Can you work these out from the model? Positions are in its coordinate system, mm. A direction names the side the tool comes from. Give positions to 0.01 mm unless a question says otherwise; leave off trailing zeros. Order: outer loops, then holes, each group sorted by start corner. A loop starts at its lowest first (then second) coordinate and runs counter-clockwise, first axis right, second up. Notation, with made-up numbers: (45.25, 19) - (93.25, 19) arc R32 cw to (93.25, 53) - close; hole circle Ø3 at (9.5, 52). An arc over 180 degrees is marked (long way). Return JSON: item names as keys, results as strings.
```python
from build123d import *

# Parameters (mm, degrees)
F0_W     = 1.4632290646
F0_H     = 3.2
F0_W_2   = 1.9813749596
F1_DEPTH = 2.4
F2_R     = 3.6
F3_R     = 0.4
F4_SIZE  = 0.4


with BuildPart() as f1:
    # F0 (on Top) → F1 (new body)
    with BuildSketch(Plane.XY):
        with BuildLine():
            Line((-1.6, 0), (1.6, 0))
            ThreePointArc((1.6, 0), (0, 1.6), (-1.6, 0))
        make_face()
        with BuildLine():
            Line((1.6, -27.8004167259), (1.6, 0))
            ThreePointArc((1.6, 0), (0, -1.6), (-1.6, 0))
            Line((-1.6, 0), (-1.6, -16.8))
            Line((-1.6, -16.8), (-1.6, -20))
            Line((-1.6, -20), (-1.6, -40))
            Line((-1.6, -40), (1.6, -40))
            Line((1.6, -40), (1.6, -31.0004167259))
            Line((1.6, -31.0004167259), (1.6, -27.8004167259))
        make_face()
        with BuildLine():
            ThreePointArc((-1.6, 0), (0, -1.6), (1.6, 0))
            Line((1.6, 0), (-1.6, 0))
        make_face()
        with Locations((2.3316145323, -29.4004167259)):
            Rectangle(F0_W, F0_H)
        with Locations((-2.5906874798, -18.4)):
            Rectangle(F0_W_2, F0_H)
        with BuildLine():
            Line((3.0632290646, -12.50463631), (3.0632290646, -27.8004167259))
            Line((3.0632290646, -27.8004167259), (3.0632290646, -31.0004167259))
            Line((3.0632290646, -31.0004167259), (6.2632290646, -31.0004167259))
            Line((6.2632290646, -31.0004167259), (6.2632290646, -12.50463631))
            ThreePointArc((6.2632290646, -12.50463631), (4.6632290646, -14.10463631), (3.0632290646, -12.50463631))
        make_face()
        with BuildLine():
            Line((-3.5813749596, -20), (-3.5813749596, -16.8))
            Line((-3.5813749596, -16.8), (-3.5813749596, -8.7620876729))
            ThreePointArc((-3.5813749596, -8.7620876729), (-5.1813749596, -10.3620876729), (-6.7813749596, -8.7620876729))
            Line((-6.7813749596, -8.7620876729), (-6.7813749596, -20))
            Line((-6.7813749596, -20), (-3.5813749596, -20))
        make_face()
        with BuildLine():
            ThreePointArc((6.2632290646, -12.50463631), (4.6632290646, -10.90463631), (3.0632290646, -12.50463631))
            Line((3.0632290646, -12.50463631), (6.2632290646, -12.50463631))
        make_face()
        with BuildLine():
            Line((6.2632290646, -12.50463631), (3.0632290646, -12.50463631))
            ThreePointArc((3.0632290646, -12.50463631), (4.6632290646, -14.10463631), (6.2632290646, -12.50463631))
        make_face()
        with BuildLine():
            ThreePointArc((-6.7813749596, -8.7620876729), (-5.1813749596, -10.3620876729), (-3.5813749596, -8.7620876729))
            Line((-3.5813749596, -8.7620876729), (-6.7813749596, -8.7620876729))
        make_face()
        with BuildLine():
            Line((-6.7813749596, -8.7620876729), (-3.5813749596, -8.7620876729))
            ThreePointArc((-3.5813749596, -8.7620876729), (-5.1813749596, -7.1620876729), (-6.7813749596, -8.7620876729))
        make_face()
    extrude(amount=F1_DEPTH)

    # F2
    f2_edges = [f1.edges().sort_by_distance(p)[0] for p in [
        (-6.781375, -20, 1.2),
        (6.263229, -31.000417, 1.2),
    ]]
    fillet(f2_edges, radius=F2_R)

    # F3
    f3_edges = [f1.edges().sort_by_distance(p)[0] for p in [
        (-3.581375, -16.8, 1.2),
        (3.063229, -27.800417, 1.2),
    ]]
    fillet(f3_edges, radius=F3_R)

    # F4
    f4_edges = [f1.edges().sort_by_distance(p)[0] for p in [
        (-3.581375, -12.581044, 2.4),
        (-3.464218, -16.682843, 2.4),
        (-5.181375, -7.162088, 2.4),
        (-2.390687, -16.8, 2.4),
        (-6.781375, -12.581044, 2.4),
        (-1.6, -8.4, 2.4),
        (-5.726959, -18.945584, 2.4),
        (0, 1.6, 2.4),
        (-2.390687, -20, 2.4),
        (1.6, -13.900208, 2.4),
        (-1.6, -30, 2.4),
        (2.131615, -27.800417, 2.4),
        (0, -40, 2.4),
        (2.946072, -27.683259, 2.4),
        (1.6, -35.500208, 2.4),
        (3.063229, -19.952527, 2.4),
        (2.131615, -31.000417, 2.4),
        (4.663229, -10.904636, 2.4),
        (5.208813, -29.946001, 2.4),
        (6.263229, -19.952527, 2.4),
        (-3.581375, -12.581044, 0),
        (-3.464218, -16.682843, 0),
        (-5.181375, -7.162088, 0),
        (-2.390687, -16.8, 0),
        (-6.781375, -12.581044, 0),
        (-1.6, -8.4, 0),
        (-5.726959, -18.945584, 0),
        (0, 1.6, 0),
        (-2.390687, -20, 0),
        (1.6, -13.900208, 0),
        (-1.6, -30, 0),
        (2.131615, -27.800417, 0),
        (0, -40, 0),
        (2.946072, -27.683259, 0),
        (1.6, -35.500208, 0),
        (3.063229, -19.952527, 0),
        (2.131615, -31.000417, 0),
        (4.663229, -10.904636, 0),
        (5.208813, -29.946001, 0),
        (6.263229, -19.952527, 0),
    ]]
    chamfer(f4_edges, length=F4_SIZE)


solid = f1.part
```
1. Suppose I cut it at B-B (z = 1.2). List the corners of the cut face in (x, y) for me, plus the area to 3 significant figures.
Checks:
{"outline": "(-6.78, -16.4) arc R3.6 ccw to (-3.18, -20) - (-1.6, -20) - (-1.6, -40) - (1.6, -40) - (1.6, -31) - (2.66, -31) arc R3.6 ccw to (6.26, -27.4) - (6.26, -12.5) arc R1.6 ccw to (3.06, -12.5) - (3.06, -27.4) arc R0.4 cw to (2.66, -27.8) - (1.6, -27.8) - (1.6, 0) arc R1.6 ccw to (-1.6, 0) - (-1.6, -16.8) - (-3.18, -16.8) arc R0.4 cw to (-3.58, -16.4) - (-3.58, -8.76) arc R1.6 ccw to (-6.78, -8.76) - close", "area": "241 mm^2"}
2. Suppose I cut it at C-C (y = -3). List the corners of the cut face in (x, z) for me, plus the area to 3 significant figures.
Checks:
{"outline": "(-1.6, 0.4) - (-1.2, 0) - (1.2, 0) - (1.6, 0.4) - (1.6, 2) - (1.2, 2.4) - (-1.2, 2.4) - (-1.6, 2) - close", "area": "7.36 mm^2"}
3. On a 3-axis mill with a long thin cutter (end or side, diameter ignored), from which of +Z, -Z, +X, -X, +Y, -Y can I reach the whole of each face in a straight line? I mean faces 5 (the face through (0, -40, 1)), 6 (the face through (3.063, -20, 1)). Say none if no direction works.
Checks:
{"face 5": "+Z, -Z, +X, -X, -Y", "face 6": "+Z, -Z, +Y"}
4. For pin 1 Ø1.3 at (y, z) = (-20, 1) entering from -X; pin 2 Ø0.8 at (x, z) = (-2.5, 1.5) entering from -Y; pin 3 Ø0.5 at (x, z) = (2.5, 1) entering from -Y, each with a flat end and sliding along its axis, tell me the tip position at first contact or that it passes through.
Checks:
{"pin 1": "x = -5.24", "pin 2": "y = -20", "pin 3": "y = -31"}
5. Suppose I cut it at A-A (y = -13.5). List the corners of the cut face in (x, z) for me.
Checks:
{"outline": "(-6.78, 0.4) - (-6.38, 0) - (-3.98, 0) - (-3.58, 0.4) - (-3.58, 2) - (-3.98, 2.4) - (-6.38, 2.4) - (-6.78, 2) - close; (-1.6, 0.4) - (-1.2, 0) - (1.2, 0) - (1.6, 0.4) - (1.6, 2) - (1.2, 2.4) - (-1.2, 2.4) - (-1.6, 2) - close; (3.06, 0.4) - (3.46, 0) - (5.86, 0) - (6.26, 0.4) - (6.26, 2) - (5.86, 2.4) - (3.46, 2.4) - (3.06, 2) - close"}
6. If I drill on L1, parallel to X at y = -15.5, z = 2.05; L2, parallel to Y at x = -3.25, z = 0.65; L3, parallel to X at y = -10, z = 1.6, over which ranges is the centre line in solid material (lowest first)? Write a range as [from, to].
Checks:
{"L1": "[-6.73, -3.63], [-1.55, 1.55], [3.11, 6.21]", "L2": "[-20, -16.79]", "L3": "[-6.78, -3.58], [-1.6, 1.6]"}
7. Thinking about a two-plate mould opening in X: for faces 1 (the face through (-5.55, -18.717, 0.114)), 2 (the face through (1, -19, 0)), 3 (the face through (-2, -16.8, 1)), 4 (the face through (6.263, -20, 1)), which applies, +X half, -X half, draft (parallel to the pull), parting line (faces both ways), or undercut?
Checks:
{"face 1": "-X half", "face 2": "draft", "face 3": "undercut", "face 4": "+X half"}
